Check sheet for the modelled part. Datum: model origin and axes. Units: mm. Face numbers are marked on the shaded views. A direction names the side the tool comes from. Round coordinates to 2 decimals unless told otherwise and drop trailing zeros. Loops run counter-clockwise (first coordinate to the right, second up) from the corner with the lowest first, then second, coordinate; pieces in that order, holes last. Notation, with made-up numbers: (-24, 66.5) - (31, 66.5) arc R16 ccw to (31, 90.5) - close; hole circle Ø6 at (43.5, 83). An arc over 180 degrees is marked (long way). Put each result on its own line as item: value. Start each with the question number.
Item 1: Section check C-C, the plane z = -97. Record the cut outline in (x, y), and give its area (3 significant figures).
Item 2: Draft check along Y on the marked faces 6, 7, 8 and 9. Enter one of: pulls with the +Y half, pulls with the -Y half, needs draft (parallel to the pull), parting line crosses it, or undercut.
Item 3: Material ranges on line 1 along Z through (x, y) = (31, 65); line 2 along Y through (x, z) = (-8, 78.5); line 3 along Y through (x, z) = (80.5, -1), recorded low to high.
Item 4: Tool access check on the marked faces 1, 2, 3, 4 and 5. Record the directions out of +Z, -Z, +X, -X, +Y, -Y that give a thin tool (end or side, any length) a straight path to the whole face; none if there is none.
Item 5: Section check A-A, the plane x = -69.5. Record the cut outline in (y, z), and give its area (3 significant figures).
Item 6: Gauge pin test, flat ends, axial feed: pin 1 Ø9 at (x, z) = (75, -14.5) entering from +Y; pin 2 Ø24 at (x, z) = (-71, 28.5) entering from +Y; pin 3 Ø1 at (y, z) = (31.5, -32.5) entering from -X. Record the tip position at first contact, or that the pin passes through.
Item 7: Section check B-B, the plane y = 92. Record the cut outline in (x, z).
Item 8: Section check D-D, the plane x = -16. Record the cut outline in (y, z), and give its area (3 significant figures).
from build123d import *

# Parameters (mm, degrees)
BOSS_EXTRUDE1_DEPTH      = 110.5
BOSS_EXTRUDE1_DEPTH_BACK = 110.5
CUT_EXTRUDE1_DEPTH       = 85.5
CUT_EXTRUDE1_DEPTH_BACK  = 85.5
SKETCH3_R                = 90
BOSS_EXTRUDE2_DEPTH      = 20
BODY_MOVE_COPY1_ANGLE    = 90


with BuildPart() as part:
    # Sketch1 → Boss-Extrude1 (new body, two sides)
    with BuildSketch(Plane(origin=(0, 0, 0), x_dir=(0, 0, -1), z_dir=(1, 0, 0))) as boss_extrude1_sk:
        with BuildLine():
            Line((-64.292863754, -51.10932545), (55.707136246, -51.10932545))
            ThreePointArc((55.707136246, -51.10932545), (69.84927187, -45.251461074), (75.707136246, -31.10932545))
            Line((75.707136246, -31.10932545), (75.707136246, 12.89067455))
            Line((75.707136246, 12.89067455), (-26.557571018, 143.789344322))
            ThreePointArc((-26.557571018, 143.789344322), (-105.517875867, 157.806043193), (-127.885671837, 80.793840961))
            Line((-127.885671837, 80.793840961), (-64.292863754, -51.10932545))
        make_face()
    extrude(amount=BOSS_EXTRUDE1_DEPTH)
    extrude(boss_extrude1_sk.sketch, amount=-BOSS_EXTRUDE1_DEPTH_BACK)

    # Sketch2 → Cut-Extrude1 (cut, two sides)
    with BuildSketch(Plane(origin=(0, 0, 0), x_dir=(0, 0, -1), z_dir=(1, 0, 0))) as cut_extrude1_sk:
        with BuildLine():
            Line((-127.885671837, 80.793840961), (-81.149808611, -16.144925076))
            ThreePointArc((-81.149808611, -16.144925076), (-21.055510127, 40.123069763), (60.857619094, 31.898033921))
            Line((60.857619094, 31.898033921), (-26.557571018, 143.789344322))
            ThreePointArc((-26.557571018, 143.789344322), (-105.517875867, 157.806043193), (-127.885671837, 80.793840961))
        make_face()
    extrude(amount=CUT_EXTRUDE1_DEPTH, mode=Mode.SUBTRACT)
    extrude(cut_extrude1_sk.sketch, amount=-CUT_EXTRUDE1_DEPTH_BACK, mode=Mode.SUBTRACT)

    # Sketch3 → Boss-Extrude2 (add)
    with BuildSketch(Plane.XZ.offset(51.10932545)):
        with Locations((0, 4.292863754)):
            Circle(SKETCH3_R)
    extrude(amount=BOSS_EXTRUDE2_DEPTH)


with BuildPart() as part_1:
    # Body-Move_Copy1: moved
    add(part.part.rotate(Axis((0, 0, 0), (0, 1, 0)), BODY_MOVE_COPY1_ANGLE))


solid = part_1.part
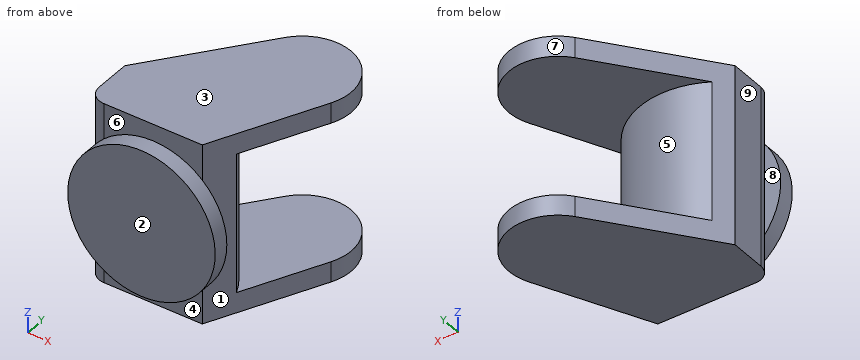
Check result:
1. outline: (-75.71, -31.11) arc R20 ccw to (-55.71, -51.11) - (64.29, -51.11) - (127.89, 80.79) arc R60 ccw to (26.56, 143.79) - (-75.71, 12.89) - close
1. area: 30,400 mm²
2. face 6: pulls with the -Y half
2. face 7: parting line crosses it
2. face 8: undercut
2. face 9: needs draft
3. line 1: -110.5 to -85.5, 85.5 to 110.5
3. line 2: -71.11 to 45.33
3. line 3: -71.11 to -51.11, -17.49 to -14.61
4. face 1: +Z, -Z, +X
4. face 2: +Z, -Z, +X, -X, -Y
4. face 3: +Z, +X, -X, +Y, -Y
4. face 4: -Z, -Y
4. face 5: +Y
5. outline: (-71.11, -51.52) - (-51.11, -51.52) - (-51.11, 51.52) - (-71.11, 51.52) - close; (-45.59, -110.5) - (20.84, -110.5) - (20.84, 110.5) - (-45.59, 110.5) - close
5. area: 16,700 mm²
6. pin 1: y = 3.2
6. pin 2: y = 32.95
6. pin 3: x = -61.56
7. outline: (-13.9, -110.5) - (131.97, -110.5) - (131.97, -85.5) - (-13.9, -85.5) - close; (-13.9, 85.5) - (131.97, 85.5) - (131.97, 110.5) - (-13.9, 110.5) - close
8. outline: (-71.11, -87.68) - (-51.11, -87.68) - (-51.11, -110.5) - (89.32, -110.5) - (89.32, -85.5) - (45.24, -85.5) - (45.24, 85.5) - (89.32, 85.5) - (89.32, 110.5) - (-51.11, 110.5) - (-51.11, 87.68) - (-71.11, 87.68) - close
8. area: 27,000 mm²
